Source: CAD feature listing. Evaluate the final solid. Frame: model axes, mm. A direction names the side the tool comes from. Round coordinates to 2 decimals unless told otherwise and drop trailing zeros. Order: outer loops, then holes, each group sorted by start corner. A loop starts at its lowest first (then second) coordinate and runs counter-clockwise, first axis right, second up. Notation, with made-up numbers: M 78.25,86 L 123.25,86 A17 cw 123.25,108 Z; hole C -5,-6.75 d4. An arc over 180 degrees is marked long. Answer as CSV lines item,"result". Start each with the question number.
Item 1: Line query: line 1 (X direction, y = -6.75, z = 0.5); line 2 (X direction, y = -6.25, z = -0.5); line 3 (Z direction, x = 0, y = -8). Output: solid intervals per line, ascending. Write a range as [from, to].
Item 2: Section query B-B on z = 25.5. State how many separate pieces and enclosed holes the cut face has, plus the area to 3 significant figures.
Item 3: Pull-direction query (Z, two-part tool) for faces 4 (the face through (-2.306, -2, -28)), 5 (the face through (-13.53, -1.7, -9.43)), 6 (the face through (-32.527, 1.565, 29.827)), 7 (the face through (33, -6.35, -30)); classes: +Z half, -Z half, draft (parallel to the pull), parting line (faces both ways), or undercut.
Item 4: First-contact query: P1, Ø0.8, axis at x = -6, z = 1.5, coming from the +Y side (3 decimals); P2, Ø1, axis at x = 2.5, y = -3, coming from the +Z side; P3, Ø2, axis at x = 0, y = -3, coming from the -Z side. Flat tips, straight axial feed; report the tip coordinate or a pass-through.
Item 5: Set-up query: faces 1 (the face through (2.182, -2, 27)), 2 (the face through (-4.6, -3.175, -4.6)), 3 (the face through (33, 0, -30)). Return all of +Z, -Z, +X, -X, +Y, -Y with unobstructed straight access to the full face (end or side cutting, diameter ignored); none if empty.
Item 6: Section query A-A on z = -35.5. Return the cut outline in (x, y) (3 decimals), plus the area to 3 significant figures.
Item 7: Section query C-C on x = -36.5. Return the cut outline in (y, z) (3 decimals).
from build123d import *

# Parameters (mm, degrees)
F0_R      = 44.1325
F1_DEPTH  = 3.175
F2_R      = 44.7675
F3_DEPTH  = 3.175
F4_R      = 44.1325
F5_DEPTH  = 3.175
F6_R      = 44.7675
F7_DEPTH  = 3.175
F8_R      = 44.7675
F9_DEPTH  = 3.175
F10_R     = 2.032
F11_DEPTH = 152.4
F13_DEPTH = 9.525
F14_R     = 6.223
F15_DEPTH = 14.732
F17_W     = 24.1837650537
F17_H     = 4.2383915279
F17_W_2   = 4.4877096079
F17_H_2   = 24.9317130074
F18_DEPTH = 25.4
F19_R     = 11.4097485145
F20_DEPTH = 25.4


with BuildPart() as f1:
    # F0 (on Front) → F1 (new body)
    with BuildSketch(Plane.XZ):
        Circle(F0_R)
    extrude(amount=-F1_DEPTH)

    # F2 (on Front) + F0 (on Front) → F3 (join)
    with BuildSketch(Plane.XZ):
        Circle(F2_R)
    with BuildSketch(Plane.XZ):
        Circle(F0_R)
    extrude(amount=F3_DEPTH)

    # F4 (on face) → F5 (join)
    with BuildSketch(Plane.XZ.offset(3.175)):
        Circle(F4_R)
    extrude(amount=F5_DEPTH)

    # F6 (on face) → F7 (join)
    with BuildSketch(Plane.XZ.offset(6.35)):
        Circle(F6_R)
    extrude(amount=F7_DEPTH)

    # F8 (on face) → F9 (join)
    with BuildSketch(Plane(origin=(0, 3.175, 0), x_dir=(-1, 0, 0), z_dir=(0, 1, 0))):
        Circle(F8_R)
    extrude(amount=F9_DEPTH)

    # F10 (on face) → F11 (cut)
    with BuildSketch(Plane.XZ.offset(9.525)):
        Circle(F10_R)
    extrude(amount=-F11_DEPTH, mode=Mode.SUBTRACT)

    # F12 (on face) → F13 (cut)
    with BuildSketch(Plane(origin=(0, 6.35, 0), x_dir=(-1, 0, 0), z_dir=(0, 1, 0))):
        Polygon((5.0649773709, -5.0970883419), (6.9466966749, 1.8378549019), (1.8817193039, 6.9349432438), (-5.0649773709, 5.0970883419), (-6.9466966749, -1.8378549019), (-1.8817193039, -6.9349432438), align=None)
    extrude(amount=-F13_DEPTH, mode=Mode.SUBTRACT)

    # F14 (on face) → F15 (cut)
    with BuildSketch(Plane.XZ.offset(9.525)):
        Circle(F14_R)
    extrude(amount=-F15_DEPTH, mode=Mode.SUBTRACT)

    # F17 (on face) → F18 (cut)
    with BuildSketch(Plane.XZ.offset(9.525)):
        with Locations((-27.6118777692, 0.0623291126)):
            Rectangle(F17_W, F17_H)
        with Locations((-0.0623329543, 27.3625557311)):
            Rectangle(F17_W_2, F17_H_2)
        with Locations((27.6118777692, 0.0623291126)):
            Rectangle(F17_W, F17_H)
        with Locations((-0.0623329543, -27.3625557311)):
            Rectangle(F17_W_2, F17_H_2)
    extrude(amount=-F18_DEPTH, mode=Mode.SUBTRACT)

    # F19 (on face) → F20 (cut)
    with BuildSketch(Plane.XZ.offset(9.525)):
        with Locations((-20.5905977637, 18.4839479625)):
            Circle(F19_R)
        with Locations((-19.6668505669, -19.046600908)):
            Circle(F19_R)
        with Locations((18.9835131168, -19.0101228654)):
            Circle(F19_R)
        with Locations((20.2279239893, 18.3876641095)):
            Circle(F19_R)
    extrude(amount=-F20_DEPTH, mode=Mode.SUBTRACT)


solid = f1.part
Results:
1,line 1,"[-44.76, -39.7], [-15.52, -6.2], [6.2, 15.52], [39.7, 44.76]"
1,line 2,"[-44.13, -39.7], [-15.52, -6.2], [6.2, 15.52], [39.7, 44.13]"
1,line 3,"[-44.77, -39.83], [-14.9, -6.22], [6.22, 14.9], [39.83, 44.77]"
2,separate pieces,"4"
2,enclosed holes,"0"
2,area,"518 mm^2"
3,face 4,"undercut"
3,face 5,"undercut"
3,face 6,"parting line"
3,face 7,"draft"
4,P1,"y = -3.175"
4,P2,"z = 44.72"
4,P3,"z = -44.77"
5,face 1,"+Y, -Y"
5,face 2,"+Y"
5,face 3,"none"
6,outline,"M -27.274,-9.525 L -2.306,-9.525 L -2.306,6.35 L -27.274,6.35 L -27.274,3.175 L -26.219,3.175 L -26.219,0 L -27.274,0 L -27.274,-3.175 L -26.219,-3.175 L -26.219,-6.35 L -27.274,-6.35 Z; M 2.182,-9.525 L 27.274,-9.525 L 27.274,-6.35 L 26.219,-6.35 L 26.219,-3.175 L 27.274,-3.175 L 27.274,0 L 26.219,0 L 26.219,3.175 L 27.274,3.175 L 27.274,6.35 L 2.182,6.35 Z"
6,area,"781 mm^2"
7,outline,"M -9.525,-25.921 L -6.35,-25.921 L -6.35,-24.808 L -3.175,-24.808 L -3.175,-25.921 L 0,-25.921 L 0,-24.808 L 3.175,-24.808 L 3.175,-25.921 L 6.35,-25.921 L 6.35,-2.057 L -9.525,-2.057 Z; M -9.525,2.182 L 6.35,2.182 L 6.35,25.921 L 3.175,25.921 L 3.175,24.808 L 0,24.808 L 0,25.921 L -3.175,25.921 L -3.175,24.808 L -6.35,24.808 L -6.35,25.921 L -9.525,25.921 Z"
